Check sheet for the modelled part. Datum: model origin and axes. Units: mm. Give positions to 0.01 mm unless a question says otherwise; leave off trailing zeros. Write each loop counter-clockwise with the first axis right and the second up, starting at its lowest first coordinate (ties: lowest second). Pieces come first, ordered by that corner, then holes. Notation, with made-up numbers: M 10,2 L 43,2 A20 cw 43,24 Z; hole C 30,-17.75 d2. An arc over 180 degrees is marked long. Use CSV: the item, a comma, the result in double quotes. Start each with the question number.
1. Depth check by flat-ended pin: P1, Ø8.5, axis at x = 393.7, y = -0.26, coming from the -Z side (3 decimals); P2, Ø3, axis at y = 33.5, z = -0.5, coming from the +X side. Enter the tip coordinate at first touch or a pass-through.
2. Cross-section at A-A, the plane x = 537.5. Enter the section's corners in (y, z) (3 decimals).
3. Cross-section at B-B, the plane z = 0.5. State how many separate pieces and enclosed holes the cut face has, and give its area (3 significant figures).
4. Scan lines: line 1 (Y direction, x = 241.3, z = -0.5); line 2 (Y direction, x = 62.5, z = 3); line 3 (X direction, y = 36.5, z = 2.25). Record each from-to range of solid material in increasing order.
5. Cross-section at C-C, the plane y = -15. Enter the section's corners in (x, z) (3 decimals).
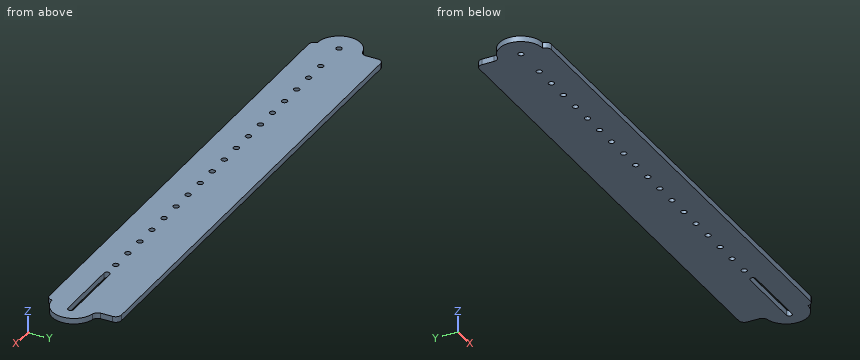
from build123d import *

# Parameters (mm, degrees)
SKETCH1_W           = 558.8
SKETCH1_H           = 25.4
SKETCH1_H_2         = 6.35
BOSS_EXTRUDE1_DEPTH = 3.175
SKETCH2_R           = 3.175
CUT_EXTRUDE1_DEPTH  = 586.064892384
FILLET1_R           = 6.35


with BuildPart() as part:
    # Sketch1 → Boss-Extrude1 (new, symmetric)
    with BuildSketch(Plane.XY):
        with Locations((279.4, 36.83)):
            Rectangle(SKETCH1_W, SKETCH1_H)
        with BuildLine():
            Line((0, -24.13), (558.8, -24.13))
            ThreePointArc((558.8, -24.13), (582.93, 0), (558.8, 24.13))
            Line((558.8, 24.13), (0, 24.13))
            ThreePointArc((0, 24.13), (-24.13, 0), (0, -24.13))
        make_face()
        with Locations((279.4, -27.305)):
            Rectangle(SKETCH1_W, SKETCH1_H_2)
    extrude(amount=BOSS_EXTRUDE1_DEPTH, both=True)

    # Sketch2 → Cut-Extrude1 (cut, through all)
    with BuildSketch(Plane.XY.offset(3.175)):
        with Locations((0.000865133, 0)):
            Circle(SKETCH2_R)
        with Locations((38.1, -0.256753551)):
            Circle(SKETCH2_R)
        with Locations((63.5, -0.256753551)):
            Circle(SKETCH2_R)
        with Locations((88.9, -0.256753551)):
            Circle(SKETCH2_R)
        with Locations((114.3, -0.256753551)):
            Circle(SKETCH2_R)
        with Locations((139.7, -0.256753551)):
            Circle(SKETCH2_R)
        with Locations((165.1, -0.256753551)):
            Circle(SKETCH2_R)
        with Locations((190.5, -0.256753551)):
            Circle(SKETCH2_R)
        with Locations((215.9, -0.256753551)):
            Circle(SKETCH2_R)
        with Locations((241.3, -0.256753551)):
            Circle(SKETCH2_R)
        with Locations((266.7, -0.256753551)):
            Circle(SKETCH2_R)
        with Locations((292.1, -0.256753551)):
            Circle(SKETCH2_R)
        with Locations((317.5, -0.256753551)):
            Circle(SKETCH2_R)
        with Locations((342.9, -0.256753551)):
            Circle(SKETCH2_R)
        with Locations((368.3, -0.256753551)):
            Circle(SKETCH2_R)
        with Locations((393.7, -0.256753551)):
            Circle(SKETCH2_R)
        with Locations((419.1, -0.256753551)):
            Circle(SKETCH2_R)
        with Locations((444.5, -0.256753551)):
            Circle(SKETCH2_R)
        with Locations((469.9, -0.256753551)):
            Circle(SKETCH2_R)
        with BuildLine():
            Line((488.95, 3.175), (565.15, 3.175))
            ThreePointArc((565.15, 3.175), (568.325, 0), (565.15, -3.175))
            Line((565.15, -3.175), (488.95, -3.175))
            ThreePointArc((488.95, -3.175), (485.775, 0), (488.95, 3.175))
        make_face()
    extrude(amount=-CUT_EXTRUDE1_DEPTH, mode=Mode.SUBTRACT)

    # Fillet1
    fillet1_edges = [part.edges().sort_by_distance(p)[0] for p in [
        (558.8, 49.53, 0),
        (558.8, 24.13, 0),
        (0, 24.13, 0),
        (0, 49.53, 0),
        (0, -30.48, 0),
        (558.8, -30.48, 0),
    ]]
    fillet(fillet1_edges, radius=FILLET1_R - 0.0001)  # a hair under: the kernel refuses the full size


solid = part.part
Worked answers:
1,P1,"stops at z = -3.175"
1,P2,"stops at x = 558.8"
2,outline,"M -30.48,-3.175 L -3.175,-3.175 L -3.175,3.175 L -30.48,3.175 Z; M 3.175,-3.175 L 49.53,-3.175 L 49.53,3.175 L 3.175,3.175 Z"
3,separate pieces,"1"
3,enclosed holes,"20"
3,area,"45,400 mm^2"
4,line 1,"y = -30.48 to -3.43, 2.92 to 49.53"
4,line 2,"y = -30.48 to -3.27, 2.76 to 49.53"
4,line 3,"x = 0 to 558.8"
5,outline,"M -18.901,-3.175 L 577.701,-3.175 L 577.701,3.175 L -18.901,3.175 Z"
